Design review of the part built by this model. Coordinates are the model's own, in mm. Face numbers are marked on the shaded views. A direction names the side the tool comes from. Round coordinates to 2 decimals unless told otherwise and drop trailing zeros. Order: outer loops, then holes, each group sorted by start corner. A loop starts at its lowest first (then second) coordinate and runs counter-clockwise, first axis right, second up.
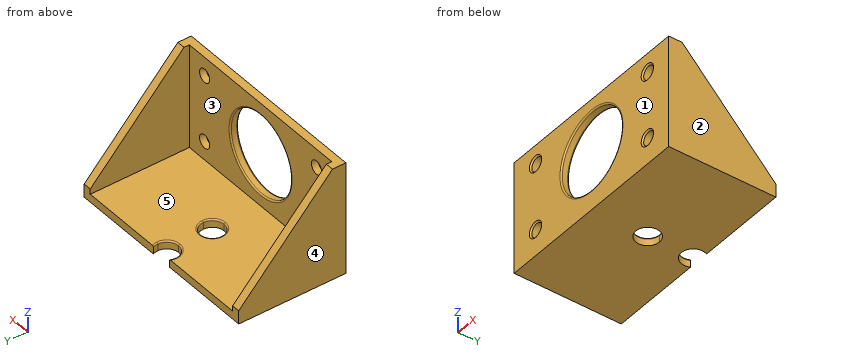
from build123d import *

# Parameters (mm, degrees)
EXTRUDE_1_DEPTH              = 3
SKETCH_2_W                   = 76
SKETCH_2_H                   = 3
EXTRUDE_2_DEPTH              = 39
CUT_EXTRUDE_1_DEPTH          = 52
CUT_EXTRUDE_2_DEPTH          = 52
EXTRUDE_3_DEPTH              = 3
HOLE_WIZARD_M6_2_D           = 5
HOLE_WIZARD_M6_2_CSINK_D     = 6.05
HOLE_WIZARD_M6_2_CSINK_ANGLE = 90
FILLET_4_R                   = 5
FILLET_5_R                   = 0.5
SKETCH_15_W                  = 76
SKETCH_15_H                  = 31.455270273
CUT_EXTRUDE_3_DEPTH          = 21


with BuildPart() as part:
    # 草图1 → 凸台-拉伸1 (new body)
    with BuildSketch(Plane.XY):
        Polygon((48, 70), (28, 70), (0, 40), (0, 0), (76, 0), (76, 40), align=None)
    extrude(amount=EXTRUDE_1_DEPTH)

    # 草图2 → 凸台-拉伸2 (add)
    with BuildSketch(Plane.XY.offset(3)):
        with Locations((38, 1.5)):
            Rectangle(SKETCH_2_W, SKETCH_2_H)
    extrude(amount=EXTRUDE_2_DEPTH)

    # 草图7 → 切除-拉伸1 (cut)
    with BuildSketch(Plane.XY.offset(3)):
        with BuildLine():
            ThreePointArc((42.4, 55), (41.111269837, 58.111269837), (38, 59.4))
            Line((38, 59.4), (38, 50.6))
            ThreePointArc((38, 50.6), (41.111269837, 51.888730163), (42.4, 55))
        make_face()
        with BuildLine():
            Line((38, 50.6), (38, 59.4))
            ThreePointArc((38, 59.4), (33.6, 55), (38, 50.6))
        make_face()
        with BuildLine():
            ThreePointArc((42.4, 38), (41.111269837, 41.111269837), (38, 42.4))
            Line((38, 42.4), (38, 33.6))
            ThreePointArc((38, 33.6), (41.111269837, 34.888730163), (42.4, 38))
        make_face()
        with BuildLine():
            Line((38, 33.6), (38, 42.4))
            ThreePointArc((38, 42.4), (33.6, 38), (38, 33.6))
        make_face()
        with BuildLine():
            ThreePointArc((42.4, 21), (41.111269837, 24.111269837), (38, 25.4))
            Line((38, 25.4), (38, 16.6))
            ThreePointArc((38, 16.6), (41.111269837, 17.888730163), (42.4, 21))
        make_face()
        with BuildLine():
            Line((38, 16.6), (38, 25.4))
            ThreePointArc((38, 25.4), (33.6, 21), (38, 16.6))
        make_face()
    extrude(amount=-CUT_EXTRUDE_1_DEPTH, mode=Mode.SUBTRACT)

    # 草图8 → 切除-拉伸2 (cut)
    with BuildSketch(Plane(origin=(0, 3, 0), x_dir=(1, 0, 0), z_dir=(0, 1, 0))):
        with BuildLine():
            ThreePointArc((23, -22.5), (38, -37.5), (53, -22.5))
            Line((53, -22.5), (23, -22.5))
        make_face()
        with BuildLine():
            Line((23, -22.5), (53, -22.5))
            ThreePointArc((53, -22.5), (38, -7.5), (23, -22.5))
        make_face()
    extrude(amount=-CUT_EXTRUDE_2_DEPTH, mode=Mode.SUBTRACT)

    # 草图10 → 凸台-拉伸3 (add)
    with BuildSketch(Plane.ZY):
        Polygon((3, 40), (5, 40), (42, 5), (42, 3), (3, 3), align=None)
    extrude_3 = extrude(amount=-EXTRUDE_3_DEPTH)

    # 镜向1: 凸台-拉伸3 across plane
    add(extrude_3.mirror(Plane(origin=(38, 0, 0), x_dir=(0, 0, 1), z_dir=(1, 0, 0))))

    # M6 螺纹孔2 (through all)
    with Locations(Plane(origin=(0, 0, 0), x_dir=(-1, 0, 0), z_dir=(0, -1, 0))):
        with Locations((-65.5, -10), (-10.5, -10), (-10.5, -35), (-65.5, -35)):
            CounterSinkHole(HOLE_WIZARD_M6_2_D / 2, HOLE_WIZARD_M6_2_CSINK_D / 2, counter_sink_angle=HOLE_WIZARD_M6_2_CSINK_ANGLE)

    # 圆角4
    fillet_4_edges = [part.edges().sort_by_distance(p)[0] for p in [
        (48, 70, 1.5),
        (28, 70, 1.5),
    ]]
    fillet(fillet_4_edges, radius=FILLET_4_R)

    # 圆角5
    fillet_5_edges = [part.edges().sort_by_distance(p)[0] for p in [
        (38, 50.6, 3),
        (38, 33.6, 3),
        (38, 16.6, 3),
        (23, 0, 22.5),
        (23, 3, 22.5),
    ]]
    fillet(fillet_5_edges, radius=FILLET_5_R)

    # 草图15 → 切除-拉伸3 (cut)
    with BuildSketch(Plane.XY.offset(3)):
        with Locations((38, 55.727635137)):
            Rectangle(SKETCH_15_W, SKETCH_15_H)
    extrude(amount=-CUT_EXTRUDE_3_DEPTH, mode=Mode.SUBTRACT)


solid = part.part
1) The part is to be moulded in two halves that separate along X. For the marked faces 1, 2 and 3, say which applies: released by +X, released by -X, zero draft, split by the parting line, or undercut.
Results:
face 1: zero draft
face 2: released by +X
face 3: undercut
2) Take a section at D-D on y = 27. Give the boundary of the cut face in (x, z), plus the area to 3 significant figures.
Results:
outline: (0, 0) - (76, 0) - (76, 18.74) - (73, 18.74) - (73, 3) - (3, 3) - (3, 18.74) - (0, 18.74) - close
area: 322 mm2
3) Take a section at C-C on x = 57.5. Give the boundary of the cut face in (y, z), plus the area to 3 significant figures.
Results:
outline: (0, 0) - (40, 0) - (40, 3) - (3, 3) - (3, 42) - (0, 42) - close
area: 237 mm2
4) To check wall thickness, follow line 1 along Z through (x, y) = (10.5, 1.5); line 2 along X through (y, z) = (1, 10); line 3 along Z through (x, y) = (65, 1). State the ranges of each line that lie inside material, in increasing order.
Results:
line 1: z = 0 to 7.5, 12.5 to 32.5, 37.5 to 42
line 2: x = 0 to 8, 13 to 29.71, 46.29 to 63, 68 to 76
line 3: z = 0 to 7.55, 12.45 to 32.55, 37.45 to 42
5) Take a section at B-B on x = 10.5. Give the boundary of the cut face in (y, z) (3 decimals), plus the area to 3 significant figures.
Results:
outline: (0, 0) - (40, 0) - (40, 3) - (3, 3) - (3, 7.5) - (0.525, 7.5) - (0, 6.975) - close; (0, 13.025) - (0.525, 12.5) - (3, 12.5) - (3, 32.5) - (0.525, 32.5) - (0, 31.975) - close; (0, 38.025) - (0.525, 37.5) - (3, 37.5) - (3, 42) - (0, 42) - close
area: 206 mm2
6) Take a section at A-A on z = 22.5. Give the boundary of the cut face in (x, y).
Results:
outline: (0, 0) - (22.5, 0) arc R0.5 ccw to (23, 0.5) - (23, 2.5) arc R0.5 ccw to (22.5, 3) - (3, 3) - (3, 23.45) - (0, 23.45) - close; (53, 0.5) arc R0.5 ccw to (53.5, 0) - (76, 0) - (76, 23.45) - (73, 23.45) - (73, 3) - (53.5, 3) arc R0.5 ccw to (53, 2.5) - close
7) Clearance check with flat-ended pins moving along their axes: P1, Ø8, axis at x = 10.5, z = 10, coming from the +Y side; P2, Ø5, axis at x = 39, y = 27, coming from the +Z side; P3, Ø3, axis at x = 65.5, z = 10, coming from the -Y side. State where each tip first meets the part, or that it passes through.
Results:
P1: stops at y = 3
P2: stops at z = 3
P3: passes through
8) For the marked faces 4 and 5, list the 3-axis set-ups (+Z, -Z, +X, -X, +Y, -Y) from which the entire face can be reached by the end or side of a thin tool; tool diameter is ignored.
Results:
face 4: +Z, -Z, -X, +Y, -Y
face 5: +Z, +Y
